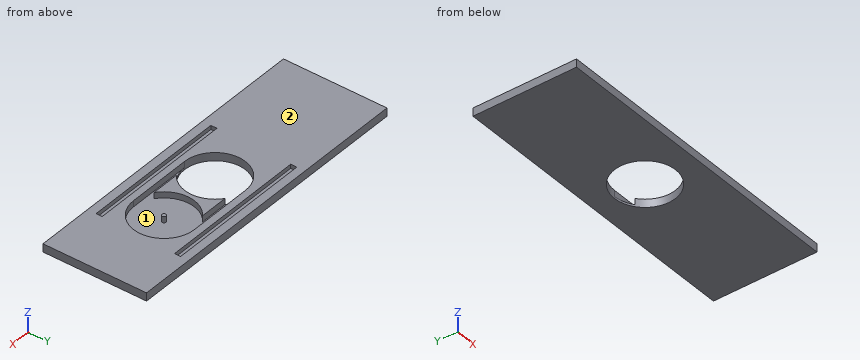
from build123d import *

# Parameters (mm, degrees)
SKETCH_W        = 75.4
SKETCH_H        = 25.5
PAD_DEPTH       = 2
SKETCH001_R     = 7.5
POCKET_DEPTH    = 2
SKETCH002_R     = 7.5
POCKET001_DEPTH = 1.5
SKETCH003_R     = 0.5
PAD001_DEPTH    = 2
SKETCH004_W     = 16
SKETCH004_H     = 1.5
POCKET002_DEPTH = 1.5
SKETCH006_W     = 36.435092
SKETCH006_H     = 1.5
SKETCH006_W_2   = 35.97442
POCKET003_DEPTH = 1


with BuildPart() as part:
    # Sketch → Pad (new body)
    with BuildSketch(Plane.XY):
        Rectangle(SKETCH_W, SKETCH_H)
    extrude(amount=PAD_DEPTH)

    # Sketch001 (on Face6 of Pad) → Pocket (cut)
    with BuildSketch(Plane.XY.offset(2)):
        Circle(SKETCH001_R)
    extrude(amount=-POCKET_DEPTH, mode=Mode.SUBTRACT)

    # Sketch002 (on Face5 of Pocket) → Pocket001 (cut)
    with BuildSketch(Plane.XY.offset(2)):
        with Locations((16, 0)):
            Circle(SKETCH002_R)
    extrude(amount=-POCKET001_DEPTH, mode=Mode.SUBTRACT)

    # Sketch003 (on Face5 of Pocket001) → Pad001 (join)
    with BuildSketch(Plane.XY.offset(2)):
        with Locations((16, 0)):
            Circle(SKETCH003_R)
    extrude(amount=-PAD001_DEPTH)

    # Sketch004 (on Face5 of Pad001) → Pocket002 (cut)
    with BuildSketch(Plane.XY.offset(2)):
        with Locations((8, 6.75)):
            Rectangle(SKETCH004_W, SKETCH004_H)
        with Locations((8, -6.75)):
            Rectangle(SKETCH004_W, SKETCH004_H)
    extrude(amount=-POCKET002_DEPTH, mode=Mode.SUBTRACT)

    # Sketch006 (on Face5 of Pocket002) → Pocket003 (cut)
    with BuildSketch(Plane.XY.offset(2)):
        with Locations((6.223254, 9.974189)):
            Rectangle(SKETCH006_W, SKETCH006_H)
        with Locations((5.741651, -9.886934)):
            Rectangle(SKETCH006_W_2, SKETCH006_H)
    extrude(amount=-POCKET003_DEPTH, mode=Mode.SUBTRACT)


solid = part.part
Source: CAD feature listing. Evaluate the final solid. Frame: model axes, mm. Face numbers are marked on the shaded views. Give positions to 0.01 mm unless a question says otherwise; leave off trailing zeros. Order: outer loops, then holes, each group sorted by start corner. A loop starts at its lowest first (then second) coordinate and runs counter-clockwise, first axis right, second up. Notation, with made-up numbers: (34.5, 50) -> (49.5, 50) arc R27 ccw to (49.5, 75) -> close; hole circle Ø9 at (41, 4). An arc over 180 degrees is marked (long way). Use a Markdown table: item, result.
1) Ray query, line 1 along Y through (x, z) = (12, 1.4); line 2 along Y through (x, z) = (-9, 1.45); line 3 along Z through (x, y) = (21.5, -3.5). Return the intervals inside material, ascending. Write a range as [from, to].
Answer list:
| item | result |
|---|---|
| line 1 | [-12.75, -10.64], [-9.14, -7.5], [7.5, 9.22], [10.72, 12.75] |
| line 2 | [-12.75, -10.64], [-9.14, 9.22], [10.72, 12.75] |
| line 3 | [0, 0.5] |
2) Section query B-B, the plane y = -5.25. Return the cut outline in (x, z), then the cut area to 3 significant figures.
Answer list:
| item | result |
|---|---|
| outline | (-37.7, 0) -> (-5.36, 0) -> (-5.36, 2) -> (-37.7, 2) -> close; (5.36, 0) -> (37.7, 0) -> (37.7, 2) -> (21.36, 2) -> (21.36, 0.5) -> (10.64, 0.5) -> (10.64, 2) -> (5.36, 2) -> close |
| area | 113 mm² |
3) Contact query for flat-ended pins moving along their axis: P1, Ø10, axis at x = 23, y = 5.5, coming from the -Z side; P2, Ø13.5, axis at x = 0, y = 0, coming from the -Z side. Output: stop coordinate, or through.
Answer list:
| item | result |
|---|---|
| P1 | z = 0 |
| P2 | through |
4) Section query A-A, the plane z = 1.3. Return the cut outline in (x, y).
Answer list:
| item | result |
|---|---|
| outline | (-37.7, -12.75) -> (37.7, -12.75) -> (37.7, 12.75) -> (-37.7, 12.75) -> close; (4.5, -6) -> (11.5, -6) arc R7.5 cw to (11.5, 6) -> (4.5, 6) arc R7.5 cw to start; circle Ø1 at (16, 0); hole (-12.25, -10.64) -> (23.73, -10.64) -> (23.73, -9.14) -> (-12.25, -9.14) -> close; hole (-11.99, 9.22) -> (24.44, 9.22) -> (24.44, 10.72) -> (-11.99, 10.72) -> close; hole (0, -7.5) -> (16, -7.5) arc R7.5 ccw to (16, 7.5) -> (0, 7.5) arc R7.5 ccw to start |
5) Mould query, pull axis X, two halves, no side actions, for the marked faces 1 and 2. Classes: +X half, -X half, draft (parallel to the pull), parting line (faces both ways), or undercut.
Answer list:
| item | result |
|---|---|
| face 1 | undercut |
| face 2 | draft |
